```python
from build123d import *

# Parameters (mm, degrees)
SKETCH1_R                      = 12.7
PART_THAT_GOES_INTO_BASE_DEPTH = 99.06
SKETCH3_R                      = 25.4
BOSS_EXTRUDE2_DEPTH            = 35.14
CUT_EXTRUDE1_START             = -75.457631354
CUT_EXTRUDE1_OUTLINE_W         = 19.304
CUT_EXTRUDE1_OUTLINE_H         = 26.758
CUT_EXTRUDE1_DEPTH             = 49.315262708
BOSS_EXTRUDE3_START            = -8.382
BOSS_EXTRUDE3_DEPTH            = 8.382
BOSS_EXTRUDE4_DEPTH            = 25.4
SKETCH7_R                      = 3.175
CUT_EXTRUDE2_DEPTH             = 12.192


# Read off the part's stored shape, not the designer's step: Cut-Extrude1
with BuildPart() as part:
    # Sketch1 → Part that goes into base (new body)
    with BuildSketch(Plane(origin=(0, 0, 0), x_dir=(1, 0, 0), z_dir=(0, 1, 0))):
        with Locations(Location((0, 0, 0), (0, 0, 270))):
            Circle(SKETCH1_R)
    extrude(amount=PART_THAT_GOES_INTO_BASE_DEPTH)

    # Sketch2 → Clip in mechanism (revolve)
    with BuildSketch(Plane.XY, mode=Mode.PRIVATE) as clip_in_mechanism_sk:
        Polygon((12.7, 62.484), (12.7, 67.564), (14.986, 67.564), align=None)
    revolve(clip_in_mechanism_sk.sketch.rotate(Axis((0, 99.06, 0), (0, -1, 0)), 90), axis=Axis((0, 99.06, 0), (0, -1, 0)))

    # Sketch3 → Boss-Extrude2 (add)
    with BuildSketch(Plane(origin=(0, 99.06, 0), x_dir=(1, 0, 0), z_dir=(0, 1, 0))):
        with Locations(Location((0, 0, 0), (0, 0, 270))):
            Circle(SKETCH3_R)
    extrude(amount=BOSS_EXTRUDE2_DEPTH)

    # Cut-Extrude1 outline → Cut-Extrude1 (cut)
    with BuildSketch(Plane(origin=(50.8, 0, 0), x_dir=(0, 0, -1), z_dir=(1, 0, 0)).offset(CUT_EXTRUDE1_START)):
        with Locations((15.748, 120.821)):
            Rectangle(CUT_EXTRUDE1_OUTLINE_W, CUT_EXTRUDE1_OUTLINE_H)
        with Locations((-15.748, 120.821)):
            Rectangle(CUT_EXTRUDE1_OUTLINE_W, CUT_EXTRUDE1_OUTLINE_H)
    extrude(amount=CUT_EXTRUDE1_DEPTH, mode=Mode.SUBTRACT)

    # Sketch5 → Boss-Extrude3 (add)
    with BuildSketch(Plane(origin=(0, 107.442, 0), x_dir=(1, 0, 0), z_dir=(0, 1, 0)).offset(BOSS_EXTRUDE3_START)):
        with BuildLine():
            Line((24.657631354, -40.386), (24.657631354, -6.096))
            ThreePointArc((24.657631354, -6.096), (0, -25.4), (-24.657631354, -6.096))
            Line((-24.657631354, -6.096), (-24.657631354, -40.386))
            Line((-24.657631354, -40.386), (24.657631354, -40.386))
        make_face()
    extrude(amount=BOSS_EXTRUDE3_DEPTH)

    # Sketch6 → Boss-Extrude4 (add)
    with BuildSketch(Plane(origin=(0, 107.442, 0), x_dir=(1, 0, 0), z_dir=(0, 1, 0))):
        Polygon((5.242487602, -34.036), (-7.020096484, -34.036), (-24.657631354, -34.036), (-24.657631354, -40.386), (24.657631354, -40.386), (24.657631354, -34.036), align=None)
    extrude(amount=BOSS_EXTRUDE4_DEPTH)

    # Sketch7 → Cut-Extrude2 (cut)
    with BuildSketch(Plane(origin=(0, 0, -6.096), x_dir=(-1, 0, 0), z_dir=(0, 0, -1))):
        with Locations(Location((0, 125.31, 0), (0, 0, 90))):
            Circle(SKETCH7_R)
    extrude(amount=-CUT_EXTRUDE2_DEPTH, mode=Mode.SUBTRACT)


solid = part.part
```
For this review, take the finished solid that the model builds, in its own axes (mm). A direction names the side the tool comes from. Round coordinates to 2 decimals unless told otherwise and drop trailing zeros. Write each loop counter-clockwise with the first axis right and the second up, starting at its lowest first coordinate (ties: lowest second). Pieces come first, ordered by that corner, then holes. Notation, with made-up numbers: (69, 26) - (99, 26) arc R20 ccw to (99, 50) - close; hole circle Ø3 at (-25.5, 49). An arc over 180 degrees is marked (long way). Answer as CSV lines item,"result". Start each with the question number.
(1) Machinability: for faces 1 (the cylindrical face through (-7.7, 30.8, -10.1)), 2 (the cylindrical face through (-7.7, 83.1, -10.1)), 3 (the flat face through (0, 107.442, 20)), which of the approach directions +Z, -Z, +X, -X, +Y, -Y give a long, thin tool a straight path to every point of the face, cutting with its end or side? Answer none if there is none.
(2) Add section B-B, the plane z = 0. State the section outline as (x, y) points (3 decimals), plus the area to 3 significant figures.
(3) Add section A-A, the plane y = 125.31. State the section outline as (x, z) points (3 decimals), plus the area to 3 significant figures.
(4) Add section D-D, the plane y = 20. State the section outline as (x, z) points.
(5) For line 1 (Z direction, x = 21, y = 112.5); line 2 (X direction, y = 125.31, z = 0) (3 decimals); line 3 (Y direction, x = 0, z = 10.5), list the stretches that pass through material, from the lowest coordinate up.
(6) For pin 1 (12 mm diameter, centred on y = 77, z = -5, fed in from -X); pin 2 (8 mm diameter, centred on x = 11, y = 118.5, fed in from -Z); pin 3 (10 mm diameter, centred on y = 25.5, z = 12.5, fed in from -X), all flat-tipped, find the tip position at first contact; note any pin that passes through.
(7) Add section C-C, the plane x = 0. State the section outline as (y, z) points (3 decimals), plus the area to 3 significant figures.
(8) Mouldability with a two-part tool opening along Y and no side actions: class faces 4 (the flat face through (0, 0, 0)), 5 (the flat face through (0, 121, 6.096)), 6 (the flat face through (0, 134.2, 0)), 7 (the cylindrical face through (-1.22, 128.24, -0.09)) as +Y half, -Y half, draft (parallel to the pull), parting line (faces both ways), or undercut.
From the geometry:
1,face 1,"-Y"
1,face 2,"none"
1,face 3,"+X, -X, +Y"
2,outline,"(-25.4, 99.06) - (-12.7, 99.06) - (-12.7, 67.564) - (-14.986, 67.564) - (-12.7, 62.484) - (-12.7, 0) - (12.7, 0) - (12.7, 62.484) - (14.986, 67.564) - (12.7, 67.564) - (12.7, 99.06) - (25.4, 99.06) - (25.4, 134.2) - (-25.4, 134.2) - close; hole circle Ø6.35 at (0, 125.31)"
2,area,"4,280 mm²"
3,outline,"(-24.658, -6.096) - (-3.175, -6.096) - (-3.175, 6.096) - (-24.658, 6.096) arc R25.4 ccw to start; (-24.658, 34.036) - (24.658, 34.036) - (24.658, 40.386) - (-24.658, 40.386) - close; (3.175, -6.096) - (24.658, -6.096) arc R25.4 ccw to (24.658, 6.096) - (3.175, 6.096) - close"
3,area,"849 mm²"
4,outline,"circle Ø25.4 at (0, 0)"
5,line 1,"z = -6.1 to 6.1, 34.04 to 40.39"
5,line 2,"x = -25.4 to -3.175, 3.175 to 25.4"
5,line 3,"y = 0 to 107.44"
6,pin 1,"stops at x = -12.7"
6,pin 2,"stops at z = -6.1"
6,pin 3,"stops at x = -10.25"
7,outline,"(0, -12.7) - (62.484, -12.7) - (67.564, -14.986) - (67.564, -12.7) - (99.06, -12.7) - (99.06, -25.4) - (107.442, -25.4) - (107.442, -6.096) - (122.135, -6.096) - (122.135, 6.096) - (107.442, 6.096) - (107.442, 34.036) - (132.842, 34.036) - (132.842, 40.386) - (99.06, 40.386) - (99.06, 12.7) - (67.564, 12.7) - (67.564, 14.986) - (62.484, 12.7) - (0, 12.7) - close; (128.485, -6.096) - (134.2, -6.096) - (134.2, 6.096) - (128.485, 6.096) - close"
7,area,"3,490 mm²"
8,face 4,"-Y half"
8,face 5,"draft"
8,face 6,"+Y half"
8,face 7,"undercut"
